from build123d import *

# Parameters (mm, degrees)
SCHIZZO1_W                  = 30
SCHIZZO1_H                  = 30
SCHIZZO1_R                  = 1.75
SCHIZZO1_R_2                = 4.25
PIASTRAAGGANCIO_DEPTH       = 4.5
SCHIZZO4_W                  = 58
SCHIZZO4_H                  = 39
BASEESC_DEPTH               = 4
SCHIZZO5_W                  = 8
SCHIZZO5_H                  = 4
APERTURAFASCETTA_DEPTH      = 57.455734873
SCHIZZO8_R                  = 1.75
CHIUSURAFORIESAGONALI_DEPTH = 2
RIMOZIONEPIASTAESC_DEPTH    = 10


with BuildPart() as part:
    # Schizzo1 → PiastraAggancio (new body)
    with BuildSketch(Plane(origin=(0, 0, 0), x_dir=(1, 0, 0), z_dir=(0, 1, 0))):
        Rectangle(SCHIZZO1_W, SCHIZZO1_H)
        with Locations(Location((6.717514421, -6.717514421, 0), (0, 0, 270))):
            Circle(SCHIZZO1_R, mode=Mode.SUBTRACT)
        with Locations(Location((-6.717514421, -6.717514421, 0), (0, 0, 270))):
            Circle(SCHIZZO1_R, mode=Mode.SUBTRACT)
        with Locations(Location((-6.717514421, 6.717514421, 0), (0, 0, 270))):
            Circle(SCHIZZO1_R, mode=Mode.SUBTRACT)
        with Locations(Location((6.717514421, 6.717514421, 0), (0, 0, 270))):
            Circle(SCHIZZO1_R, mode=Mode.SUBTRACT)
        with Locations(Location((0, 0, 0), (0, 0, 270))):
            Circle(SCHIZZO1_R_2, mode=Mode.SUBTRACT)
        Polygon((12.6, -3.031088913), (14.35, 0), (12.6, 3.031088913), (9.1, 3.031088913), (7.35, 0), (9.1, -3.031088913), align=None, mode=Mode.SUBTRACT)
        Polygon((-3.5, -10), (-1.75, -13.031088913), (1.75, -13.031088913), (3.5, -10), (1.75, -6.968911087), (-1.75, -6.968911087), align=None, mode=Mode.SUBTRACT)
        Polygon((-14.35, 0), (-12.6, -3.031088913), (-9.1, -3.031088913), (-7.35, 0), (-9.1, 3.031088913), (-12.6, 3.031088913), align=None, mode=Mode.SUBTRACT)
        Polygon((1.75, 6.968911087), (3.5, 10), (1.75, 13.031088913), (-1.75, 13.031088913), (-3.5, 10), (-1.75, 6.968911087), align=None, mode=Mode.SUBTRACT)
    extrude(amount=PIASTRAAGGANCIO_DEPTH)

    # Schizzo4 → BaseESC (add)
    with BuildSketch(Plane(origin=(15, 0, 0), x_dir=(0, 0, -1), z_dir=(1, 0, 0))):
        with Locations((0, -15)):
            Rectangle(SCHIZZO4_W, SCHIZZO4_H)
    extrude(amount=BASEESC_DEPTH)

    # Schizzo5 → AperturaFascetta (cut, through all)
    with BuildSketch(Plane(origin=(19, 0, 0), x_dir=(0, 0, -1), z_dir=(1, 0, 0))):
        with Locations((-21, -0.5)):
            Rectangle(SCHIZZO5_W, SCHIZZO5_H)
        with Locations((21, -0.5)):
            Rectangle(SCHIZZO5_W, SCHIZZO5_H)
        with Locations((21, -29.5)):
            Rectangle(SCHIZZO5_W, SCHIZZO5_H)
        with Locations((-21, -29.5)):
            Rectangle(SCHIZZO5_W, SCHIZZO5_H)
    extrude(amount=-APERTURAFASCETTA_DEPTH, mode=Mode.SUBTRACT)

    # Schizzo7 → SvasaturaVitiInferiori (revolve, cut)
    with BuildSketch(Plane.XY.offset(6.717514421), mode=Mode.PRIVATE) as svasaturavitiinferiori_sk:
        Polygon((-9.217514421, 0), (-8.467514421, 2), (-6.717514421, 2), (-6.717514421, 0), align=None)
    svasaturavitiinferiori = revolve(svasaturavitiinferiori_sk.sketch.rotate(Axis((-6.717514421, 2, 6.717514421), (0, -1, 0)), 270), axis=Axis((-6.717514421, 2, 6.717514421), (0, -1, 0)), mode=Mode.SUBTRACT)

    # SvasaturaVitiInferiori2: SvasaturaVitiInferiori across plane
    add(svasaturavitiinferiori.mirror(Plane(origin=(0, 0, 0), x_dir=(0, 0, 1), z_dir=(1, 0, 0))), mode=Mode.SUBTRACT)

    # SvasaturaVitiInferiori3: SvasaturaVitiInferiori across plane
    add(svasaturavitiinferiori.mirror(Plane.XY), mode=Mode.SUBTRACT)

    # SvasaturaVitiInferiori3 copy 1 sketch → SvasaturaVitiInferiori3 copy 1 (revolve, cut)
    with BuildSketch(Plane(origin=(0, 0, -6.717514421), x_dir=(-1, 0, 0), z_dir=(0, 0, -1))):
        Polygon((-9.217514421, 0), (-8.467514421, 2), (-6.717514421, 2), (-6.717514421, 0), align=None)
    revolve(axis=Axis((6.717514421, 2, -6.717514421), (0, -1, 0)), mode=Mode.SUBTRACT)

    # Schizzo8 → ChiusuraForiEsagonali (add)
    # profile 1 of 4: a face of its own
    with BuildSketch(Plane.XZ):
        Polygon((1.75, -13.031088913), (3.5, -10), (1.75, -6.968911087), (-1.75, -6.968911087), (-3.5, -10), (-1.75, -13.031088913), align=None)
        with Locations(Location((0, -10, 0), (0, 0, 270))):
            Circle(SCHIZZO8_R, mode=Mode.SUBTRACT)
    # profile 2 of 4: a face of its own
    with BuildSketch(Plane.XZ):
        Polygon((12.6, 3.031088913), (9.1, 3.031088913), (7.35, 0), (9.1, -3.031088913), (12.6, -3.031088913), (14.35, 0), align=None)
        with Locations(Location((10.85, 0, 0), (0, 0, 270))):
            Circle(SCHIZZO8_R, mode=Mode.SUBTRACT)
    # profile 3 of 4: a face of its own
    with BuildSketch(Plane.XZ):
        Polygon((-1.75, 13.031088913), (-3.5, 10), (-1.75, 6.968911087), (1.75, 6.968911087), (3.5, 10), (1.75, 13.031088913), align=None)
        with Locations(Location((0, 10, 0), (0, 0, 270))):
            Circle(SCHIZZO8_R, mode=Mode.SUBTRACT)
    # profile 4 of 4: a face of its own
    with BuildSketch(Plane.XZ):
        Polygon((-14.35, 0), (-12.6, -3.031088913), (-9.1, -3.031088913), (-7.35, 0), (-9.1, 3.031088913), (-12.6, 3.031088913), align=None)
        with Locations(Location((-10.85, 0, 0), (0, 0, 270))):
            Circle(SCHIZZO8_R, mode=Mode.SUBTRACT)
    extrude(amount=-CHIUSURAFORIESAGONALI_DEPTH)

    # Schizzo9 → RimozionePiastaESC (cut)
    with BuildSketch(Plane.ZY.offset(-15)):
        Polygon((-15, 0), (-15, -3), (15, -3), (15, 0), (15, 4.5), (29, 4.5), (29, -34.5), (-29, -34.5), (-29, 4.5), (-15, 4.5), align=None)
    extrude(amount=-RIMOZIONEPIASTAESC_DEPTH, mode=Mode.SUBTRACT)


solid = part.part
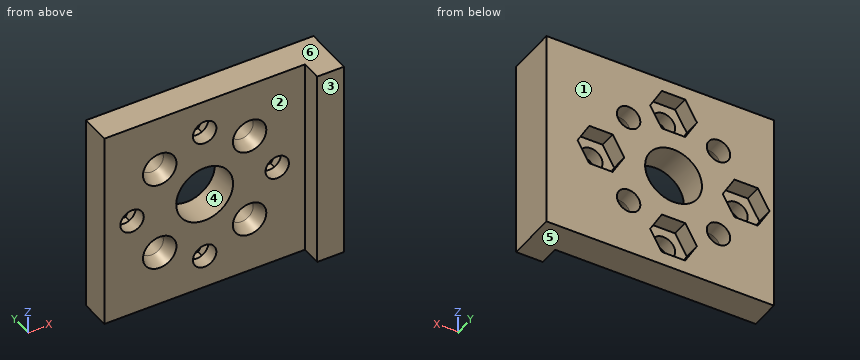
Can you work these out from the model? Positions are in its coordinate system, mm. Face numbers are marked on the shaded views. A direction names the side the tool comes from. Round coordinates to 2 decimals unless told otherwise and drop trailing zeros. Write each loop counter-clockwise with the first axis right and the second up, starting at its lowest first coordinate (ties: lowest second). Pieces come first, ordered by that corner, then holes. Notation, with made-up numbers: M 85,70 L 133,70 A24 ccw 133,107 Z; hole C 30.5,7 d5. An arc over 180 degrees is marked long. Use a Markdown table: item, result.
Item 1: I want a section at A-A (x = -10.85). List the corners of the cut face in (y, z) for me.
Found:
| item | result |
|---|---|
| outline | M 0,-15 L 4.5,-15 L 4.5,-3.03 L 2,-3.03 L 2,-1.75 L 0,-1.75 Z; M 0,1.75 L 2,1.75 L 2,3.03 L 4.5,3.03 L 4.5,15 L 0,15 Z |
Item 2: Which directions (+Z, -Z, +X, -X, +Y, -Y) give clear straight access to the entire face, cutting with the end or side of a thin tool? Please do the marked faces 1 and 2.
Found:
| item | result |
|---|---|
| face 1 | +Z, -Z, +X, -X, +Y |
| face 2 | +Z, -Z, -X, -Y |
Item 3: We'd pull the mould along Z, two halves only. Please class the marked faces 3, 4, 5 and 6: released by +Z, released by -Z, zero draft, split by the parting line, or undercut.
Found:
| item | result |
|---|---|
| face 3 | zero draft |
| face 4 | undercut |
| face 5 | released by -Z |
| face 6 | released by +Z |
Item 4: I want a section at D-D (y = 0.5). State how many separate pieces and enclosed holes the cut face has, and give its area (3 significant figures).
Found:
| item | result |
|---|---|
| separate pieces | 1 |
| enclosed holes | 9 |
| area | 858 mm2 |
Item 5: If I drill on line 1 along X through (y, z) = (1.1, 10); line 2 along Z through (x, y) = (-10, 3.25); line 3 along Z through (x, y) = (8, 2.75), over which ranges is the centre line in solid material (lowest first)? Write a range as [from, to].
Found:
| item | result |
|---|---|
| line 1 | x = [-15, -1.75], [1.75, 19] |
| line 2 | z = [-15, -3.03], [3.03, 15] |
| line 3 | z = [-15, -7.91], [-5.53, -1.13], [1.13, 5.53], [7.91, 15] |
Item 6: I want a section at C-C (x = 1). List the corners of the cut face in (y, z) for me, and give its area (3 significant figures).
Found:
| item | result |
|---|---|
| outline | M 0,-15 L 4.5,-15 L 4.5,-13.03 L 2,-13.03 L 2,-11.44 L 0,-11.44 Z; M 0,-8.56 L 2,-8.56 L 2,-6.97 L 4.5,-6.97 L 4.5,-4.13 L 0,-4.13 Z; M 0,4.13 L 4.5,4.13 L 4.5,6.97 L 2,6.97 L 2,8.56 L 0,8.56 Z; M 0,11.44 L 2,11.44 L 2,13.03 L 4.5,13.03 L 4.5,15 L 0,15 Z |
| area | 56.0 mm2 |
Item 7: I want a section at B-B (z = -11). List the corners of the cut face in (x, y) for me, and give its area (3 significant figures).
Found:
| item | result |
|---|---|
| outline | M -15,0 L -1.44,0 L -1.44,2 L -2.92,2 L -2.92,4.5 L -15,4.5 Z; M 1.44,0 L 15,0 L 15,-3 L 19,-3 L 19,4.5 L 2.92,4.5 L 2.92,2 L 1.44,2 Z |
| area | 145 mm2 |
Item 8: For pin 1 Ø5.5 at (x, z) = (10.85, 0) entering from +Y; pin 2 Ø3.5 at (y, z) = (-2, 3) entering from -X; pin 3 Ø4.5 at (x, z) = (0, -10) entering from -Y, each with a flat end and sliding along its axis, tell me the tip position at first contact or that it passes through.
Found:
| item | result |
|---|---|
| pin 1 | stops at y = 2 |
| pin 2 | stops at x = 15 |
| pin 3 | stops at y = 0 |
